Design review of the part shown in the three views and the two pictorial views. Dimensions are in mm from the part's minimum x, y and z. A direction names the side the tool comes from. Round coordinates to 2 decimals unless told otherwise and drop trailing zeros. Write each loop counter-clockwise with the first axis right and the second up, starting at its lowest first coordinate (ties: lowest second). Pieces come first, ordered by that corner, then holes. Notation, with made-up numbers: (19.5, 86.25) - (59.5, 86.25) arc R27 cw to (59.5, 110.25) - close; hole circle Ø9 at (51, -30). An arc over 180 degrees is marked (long way). Use one line per item in the form item = value.
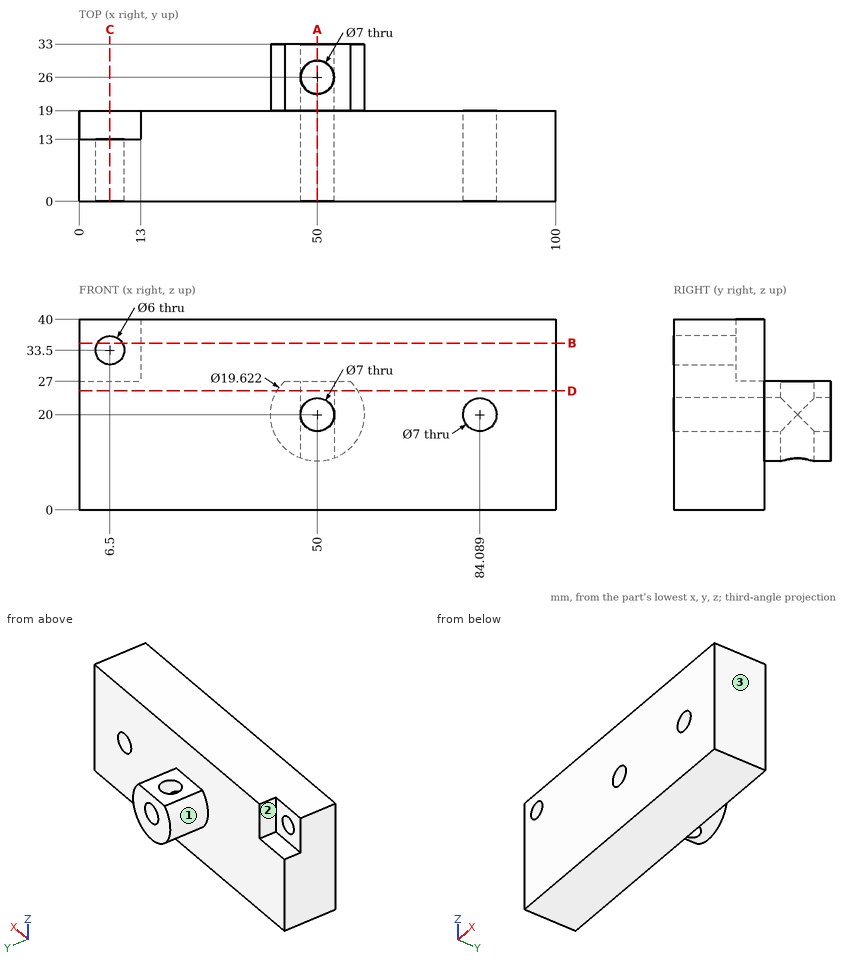
Q1. We need section A-A on x = 50. Write out the cut boundary in (y, z), then the cut area to 3 significant figures.
Calculated:
outline = (0, 0) - (19, 0) - (19, 10.19) - (22.5, 10.19) - (22.5, 16.5) - (0, 16.5) - close; (0, 23.5) - (22.5, 23.5) - (22.5, 27) - (19, 27) - (19, 40) - (0, 40) - close; (29.5, 10.19) - (33, 10.19) - (33, 16.5) - (29.5, 16.5) - close; (29.5, 23.5) - (33, 23.5) - (33, 27) - (29.5, 27) - close
area = 696 mm2
Q2. We need section C-C on x = 6.5. Write out the cut boundary in (y, z).
Calculated:
outline = (0, 0) - (19, 0) - (19, 27) - (13, 27) - (13, 30.5) - (0, 30.5) - close; (0, 36.5) - (13, 36.5) - (13, 40) - (0, 40) - close
Q3. We need section B-B on z = 35. Write out the cut boundary in (x, y), then the cut area to 3 significant figures.
Calculated:
outline = (0, 0) - (3.9, 0) - (3.9, 13) - (0, 13) - close; (9.1, 0) - (100, 0) - (100, 19) - (13, 19) - (13, 13) - (9.1, 13) - close
area = 1,750 mm2
Q4. For P1, Ø15, axis at x = 52.5, y = 27, coming from the +Z side; P2, Ø1.8, axis at y = 16, z = 33.5, coming from the -X side; P3, Ø1.5, axis at y = 24.5, z = 20, coming from the +X side, all flat-tipped, find the tip position at first contact; note any pin that passes through.
Calculated:
P1 = 27
P2 = 13
P3 = 59.81
Q5. We need section D-D on z = 25. Write out the cut boundary in (x, y), then the cut area to 3 significant figures.
Calculated:
outline = (0, 0) - (100, 0) - (100, 19) - (58.44, 19) - (58.44, 33) - (41.56, 33) - (41.56, 19) - (0, 19) - close; hole circle Ø7 at (50, 26)
area = 2,100 mm2
Q6. Machinability: for the marked faces 1, 2 and 3, which of the approach directions +Z, -Z, +X, -X, +Y, -Y give a long, thin tool a straight path to every point of the face, cutting with its end or side? Answer none if there is none.
Calculated:
face_1 = +Y
face_2 = +Z, -X, +Y
face_3 = +Z, -Z, +X, +Y, -Y
Q7. To check wall thickness, follow line 1 along X through (y, z) = (27.5, 20); line 2 along Z through (x, y) = (6.5, 9.25); line 3 along X through (y, z) = (24.5, 21). State the ranges of each line that lie inside material, in increasing order. Write a range as from..to.
Calculated:
line_1 = 40.19..46.5, 53.5..59.81
line_2 = 0..30.5, 36.5..40
line_3 = 40.24..46.65, 53.35..59.76
